Geometry: final body of the model. Coordinates: model frame, mm. Face numbers are marked on the shaded views. A direction names the side the tool comes from. Round coordinates to 2 decimals unless told otherwise and drop trailing zeros. Loops run counter-clockwise (first coordinate to the right, second up) from the corner with the lowest first, then second, coordinate; pieces in that order, holes last. Notation, with made-up numbers: (-1.5, 47.5) -> (53.5, 47.5) arc R18 cw to (53.5, 51.5) -> close; hole circle Ø10 at (80, 29.25). An arc over 180 degrees is marked (long way). Answer in a Markdown table with one row per item.
Autodesk Inventor part; units mm, degrees
ref_plane "YZ Plane" through (0, 0, 0) normal (1, 0, 0) x (0, 1, 0)
ref_plane "XZ Plane" through (0, 0, 0) normal (0, 1, 0) x (-1, 0, 0)
ref_plane "XY Plane" through (0, 0, 0) normal (0, 0, 1) x (1, 0, 0)
sketch "Sketch1" plane through (0, 0, 0) normal (0, 0, 1) x (1, 0, 0)
  line L0 (0, 0) -> (40.12, 0)
  line L1 (40.12, 0) -> (40.12, 58.1)
  line L2 (40.12, 58.1) -> (0, 58.1)
  line L3 (0, 58.1) -> (0, 0)
  circle A0 centre (20.06, 20.2) radius 4
  line L4 (6.06, 49.5) -> (34.06, 49.5) construction
  line L5 (34.06, 49.5) -> (34.06, 9.5) construction
  line L6 (34.06, 9.5) -> (6.06, 9.5) construction
  line L7 (6.06, 9.5) -> (6.06, 49.5) construction
  circle A1 centre (6.06, 49.5) radius 2
  circle A2 centre (34.06, 49.5) radius 2
  circle A3 centre (34.06, 9.5) radius 2
  circle A4 centre (6.06, 9.5) radius 2
  point P0 (20.06, 58.1)
  point P1 (20.06, 49.5)
  dimension "d0" = 40.12
  dimension "d1" = 58.1
  dimension "d2" = 8
  dimension "d3" = 37.9
  dimension "d4" = 28
  dimension "d5" = 40
  dimension "d6" = 8.6
  dimension "d7" = 4
  dimension "d8" = 4
  dimension "d9" = 4
  dimension "d10" = 4
extrude "Extrusion1" add sketch "Sketch1" along normal blind 27
sketch "Sketch2" plane through (0, 0, 27) normal (0, 0, 1) x (1, 0, 0)
  circle A0 centre (6.06, 49.5) radius 2
  circle A1 centre (34.06, 49.5) radius 2
  circle A2 centre (20.06, 20.2) radius 4
  circle A3 centre (34.06, 9.5) radius 2
  circle A4 centre (6.06, 9.5) radius 2
  circle A5 centre (6.06, 49.5) radius 2
  circle A6 centre (6.06, 49.5) radius 3.9
  circle A7 centre (34.06, 9.5) radius 2
  circle A8 centre (34.06, 9.5) radius 3.9
  circle A9 centre (34.06, 49.5) radius 2
  circle A10 centre (34.06, 49.5) radius 3.9
  circle A11 centre (6.06, 9.5) radius 3.9
  circle A12 centre (20.06, 20.2) radius 9.375
  point P0 (0, 0)
  dimension "d13" = 7.8
  dimension "d14" = 7.8
  dimension "d15" = 7.8
  dimension "d16" = 7.8
  dimension "d17" = 18.75
extrude "Extrusion2" add sketch "Sketch2" along normal blind 2
sketch "Sketch3" plane through (0, 0, 27) normal (0, 0, 1) x (1, 0, 0)
  circle A0 centre (20.06, 20.2) radius 9.375
  circle A1 centre (20.06, 20.2) radius 4
  point P0 (0, 0)
extrude "Extrusion3" add sketch "Sketch3" along normal blind 3.5
sketch "Sketch4" plane through (0, 0, 0) normal (0, 0, -1) x (-1, 0, 0)
  circle A0 centre (-20.06, 20.2) radius 9.375
  circle A1 centre (-20.06, 20.2) radius 4
  point P0 (0, 0)
extrude "Extrusion4" add sketch "Sketch4" along normal blind 3.5
sketch "Sketch5" plane through (20.06, 20.2, -3.5) normal (0, 0, -1) x (-1, 0, 0)
  circle A0 centre (0, 0) radius 9.375
  point P0 (20.06, -20.2)
extrude "Extrusion5" add sketch "Sketch5" against normal up to surface (34 mm away) from surface at 0
sketch "Sketch6" plane through (20.06, 20.2, 30.5) normal (0, 0, 1) x (1, 0, 0)
  circle A0 centre (0, 0) radius 4
  circle A1 centre (0, 0) radius 9.375
  point P0 (-20.06, -20.2)
  dimension "d26" = 8
extrude "Extrusion6" add sketch "Sketch6" along normal blind 16 contours A0
sketch "Sketch7" plane through (20.06, 20.2, 46.5) normal (0, 0, 1) x (1, 0, 0)
  line L0 (-2.6458, 3) -> (2.6458, 3)
  circle A0 centre (0, 0) radius 4
  arc A1 (-2.6458, 3) -> (2.6458, 3) centre (0, 0) ccw
  point P0 (-20.06, -20.2)
  point P1 (0, 3)
  dimension "d29" = 7
extrude "Extrusion7" cut sketch "Sketch7" against normal blind 13 contours A0 L0 picked at (0.5822, 3.4764)
sketch "Sketch8" plane through (0, 58.1, 0) normal (0, 1, 0) x (1, 0, 0)
  circle A0 centre (20.06, -9.5) radius 15.5
  line L0 (40.12, -27) -> (0, -27)
  line L1 (40.12, 0) -> (40.12, -27)
  line L2 (40.12, -13.5) -> (0, -13.5)
  point P0 (0, 0)
  point P1 (20.06, -27)
  point P2 (20.06, -13.5)
  dimension "d32" = 31
  dimension "d34" = 4
extrude "Extrusion8" add sketch "Sketch8" along normal blind 57.2
sketch "Sketch10" plane through (20.06, 115.3, 9.5) normal (0, 1, 0) x (1, 0, 0)
  circle A0 centre (0, 0) radius 6
  circle A1 centre (0, 0) radius 15.5
  point P0 (-20.06, 9.5)
  dimension "d37" = 12
extrude "Extrusion9" add sketch "Sketch10" along normal blind 2 contours A0
sketch "Sketch11" plane through (20.06, 115.3, 9.5) normal (0, 1, 0) x (1, 0, 0)
  circle A0 centre (0, 0) radius 15.5
  circle A1 centre (0, 0) radius 15.4
  point P0 (-20.06, 9.5)
  dimension "d40" = 0.1
extrude "Extrusion10" cut sketch "Sketch11" against normal blind 3
sketch "Sketch12" plane through (0, 58.1, 27) normal (0, 1, 0) x (1, 0, 0)
  circle A0 centre (20.06, 17.5) radius 15.4
  circle A1 centre (20.06, 17.5) radius 15.5
  point P0 (0, 27)
extrude "Extrusion11" cut sketch "Sketch12" along normal blind 3
sketch "Sketch13" plane through (0, 0, 0) normal (0, 0, -1) x (-1, 0, 0)
  circle A0 centre (-6.06, 49.5) radius 3.9
  circle A1 centre (-34.06, 49.5) radius 3.9
  circle A2 centre (-34.06, 9.5) radius 3.9
  circle A3 centre (-6.06, 9.5) radius 3.9
  circle A4 centre (-6.06, 9.5) radius 2
  circle A5 centre (-6.06, 49.5) radius 2
  circle A6 centre (-34.06, 49.5) radius 2
  circle A7 centre (-34.06, 9.5) radius 2
  point P0 (0, 0)
extrude "Extrusion12" add sketch "Sketch13" along normal blind 2
fillet "Fillet1" radius 2 4 edges at (40.12, 58.1, 13.5) (0, 58.1, 13.5) (0, 0, 13.5) (40.12, 0, 13.5)
properties part number "TS-40GZ495" material "Stainless Steel"
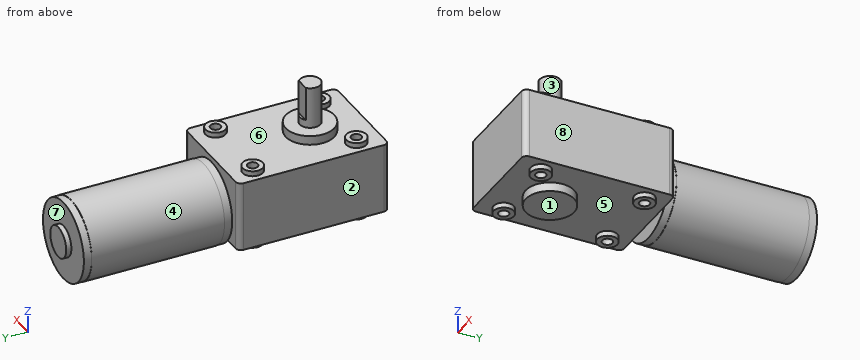
Item 1: Draft query along X for the marked faces 6, 7 and 8. Return one class per face: pulls with the +X half, pulls with the -X half, needs draft (parallel to the pull), parting line crosses it, or undercut.
Answer:
| item | result |
|---|---|
| face 6 | undercut |
| face 7 | needs draft |
| face 8 | pulls with the +X half |
Item 2: Cut plane B-B (z = 9.5). Output: boundary loops of the cut face in (x, y), then the cut area to 3 significant figures.
Answer:
| item | result |
|---|---|
| outline | (0, 2) arc R2 ccw to (2, 0) -> (38.12, 0) arc R2 ccw to (40.12, 2) -> (40.12, 56.1) arc R2 ccw to (38.12, 58.1) -> (35.46, 58.1) -> (35.46, 61.1) -> (35.56, 61.1) -> (35.56, 112.3) -> (35.46, 112.3) -> (35.46, 115.3) -> (26.06, 115.3) -> (26.06, 117.3) -> (14.06, 117.3) -> (14.06, 115.3) -> (4.66, 115.3) -> (4.66, 112.3) -> (4.56, 112.3) -> (4.56, 61.1) -> (4.66, 61.1) -> (4.66, 58.1) -> (2, 58.1) arc R2 ccw to (0, 56.1) -> close; hole circle Ø4 at (6.06, 9.5); hole circle Ø4 at (6.06, 49.5); hole circle Ø4 at (34.06, 9.5); hole circle Ø4 at (34.06, 49.5) |
| area | 4,070 mm² |
Item 3: Reachability of the marked faces 1, 2, 3, 4 and 5 from +Z, -Z, +X, -X, +Y, -Y: full face, straight path, thin tool, end or side. Return the list, or none.
Answer:
| item | result |
|---|---|
| face 1 | -Z, +X, -X, -Y |
| face 2 | +Z, -Z, -X, +Y, -Y |
| face 3 | +Z |
| face 4 | +Y |
| face 5 | -Z |
Item 4: Cut plane C-C (y = 20.2). Output: boundary loops of the cut face in (x, z) (3 decimals).
Answer:
| item | result |
|---|---|
| outline | (0, 0) -> (10.685, 0) -> (10.685, -3.5) -> (29.435, -3.5) -> (29.435, 0) -> (40.12, 0) -> (40.12, 27) -> (29.435, 27) -> (29.435, 30.5) -> (24.06, 30.5) -> (24.06, 46.5) -> (16.06, 46.5) -> (16.06, 30.5) -> (10.685, 30.5) -> (10.685, 27) -> (0, 27) -> close |
Item 5: Cut plane A-A (y = 49.5). Output: boundary loops of the cut face in (x, z), then the cut area to 3 significant figures.
Answer:
| item | result |
|---|---|
| outline | (0, 0) -> (2.16, 0) -> (2.16, -2) -> (4.06, -2) -> (4.06, 29) -> (2.16, 29) -> (2.16, 27) -> (0, 27) -> close; (8.06, -2) -> (9.96, -2) -> (9.96, 0) -> (30.16, 0) -> (30.16, -2) -> (32.06, -2) -> (32.06, 29) -> (30.16, 29) -> (30.16, 27) -> (9.96, 27) -> (9.96, 29) -> (8.06, 29) -> close; (36.06, -2) -> (37.96, -2) -> (37.96, 0) -> (40.12, 0) -> (40.12, 27) -> (37.96, 27) -> (37.96, 29) -> (36.06, 29) -> close |
| area | 898 mm² |
Item 6: Line query: probe 1 along Y at (x, z) = (34.06, -1.35); probe 2 along Y at (x, z) = (6.06, 7.5); probe 3 along X at (y, z) = (49.5, 7.75). Output: solid intervals per line, ascending. Write a range as [from, to].
Answer:
| item | result |
|---|---|
| probe 1 | y = [5.6, 7.5], [11.5, 13.4], [45.6, 47.5], [51.5, 53.4] |
| probe 2 | y = [0, 7.5], [11.5, 47.5], [51.5, 115.3] |
| probe 3 | x = [0, 4.06], [8.06, 32.06], [36.06, 40.12] |
Item 7: Pin query (flat end, axial travel): pin 1 Ø3 at (y, z) = (53.5, 31.5) entering from +X; pin 2 Ø9.5 at (x, y) = (22.5, 17.5) entering from -Z; pin 3 Ø2 at (x, z) = (6.5, 25) entering from +Y; pin 4 Ø6 at (x, y) = (34.5, 8.5) entering from -Z. Return the tip coordinate at first contact, or that it passes through.
Answer:
| item | result |
|---|---|
| pin 1 | passes through |
| pin 2 | stops at z = -3.5 |
| pin 3 | stops at y = 58.1 |
| pin 4 | stops at z = -2 |
